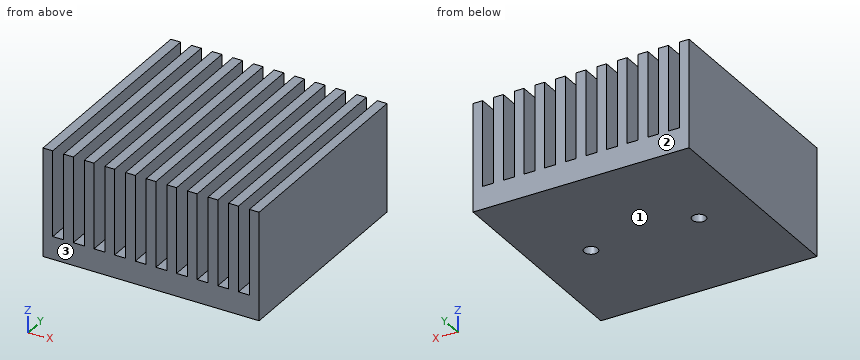
```python
from build123d import *

# Parameters (mm, degrees)
ESQUISSE1_W                = 40
ESQUISSE1_H                = 40
BOSS_EXTRU_1_DEPTH         = 4.2
ESQUISSE2_W                = 1.8
ESQUISSE2_H                = 15.8
BOSS_EXTRU_2_DEPTH         = 40
R_P_TITION_LIN_AIRE1_COUNT = 11
R_P_TITION_LIN_AIRE1_PITCH = 3.82
ESQUISSE3_R                = 1.25
ENL_V_MAT_EXTRU_1_DEPTH    = 10


with BuildPart() as part:
    # Esquisse1 → Boss.-Extru.1 (new body)
    with BuildSketch(Plane.XY):
        with Locations((20, 20)):
            Rectangle(ESQUISSE1_W, ESQUISSE1_H)
    extrude(amount=BOSS_EXTRU_1_DEPTH)

    # Esquisse2 → Boss.-Extru.2 (add)
    with BuildSketch(Plane.XZ):
        with Locations((0.9, 12.1)):
            Rectangle(ESQUISSE2_W, ESQUISSE2_H)
    boss_extru_2 = extrude(amount=-BOSS_EXTRU_2_DEPTH)

    # Répétition linéaire1: Boss.-Extru.2 ×11
    with Locations(*[(i * R_P_TITION_LIN_AIRE1_PITCH, 0, 0) for i in range(1, R_P_TITION_LIN_AIRE1_COUNT)]):
        add(boss_extru_2)

    # Esquisse3 → Enlèv. mat.-Extru.1 (cut)
    with BuildSketch(Plane(origin=(0, 0, 0), x_dir=(-1, 0, 0), z_dir=(0, 0, -1))):
        with Locations((-30, 20)):
            Circle(ESQUISSE3_R)
        with Locations((-10, 20)):
            Circle(ESQUISSE3_R)
    extrude(amount=-ENL_V_MAT_EXTRU_1_DEPTH, mode=Mode.SUBTRACT)


solid = part.part
```
The model under review builds one solid part; all positions refer to its coordinate system, in mm. Face numbers are marked on the shaded views. Give positions to 0.01 mm unless a question says otherwise; leave off trailing zeros. Loops run counter-clockwise (first coordinate to the right, second up) from the corner with the lowest first, then second, coordinate; pieces in that order, holes last. Notation, with made-up numbers: (4, 58.25) - (57, 58.25) arc R14 ccw to (57, 71.25) - close; hole circle Ø3 at (61, 21.25). An arc over 180 degrees is marked (long way). Answer as a JSON object with one key per item and string values.
Q1. Add section A-A on x = 10. State the section outline as (y, z) points, plus the area to 4 significant figures.
Worked out:
{"outline": "(0, 0) - (18.75, 0) - (18.75, 4.2) - (0, 4.2) - close; (21.25, 0) - (40, 0) - (40, 4.2) - (21.25, 4.2) - close", "area": "157.5 mm^2"}
Q2. To check wall thickness, follow line 1 along Z through (x, y) = (15, 28.5); line 2 along Y through (x, z) = (30, 3.5); line 3 along Y through (x, z) = (31, 5.5). State the ranges of each line that lie inside material, in increasing order.
Worked out:
{"line 1": "z = 0 to 4.2", "line 2": "y = 0 to 18.75, 21.25 to 40", "line 3": "y = 0 to 19.25, 20.75 to 40"}
Q3. Mouldability with a two-part tool opening along Y and no side actions: class the marked faces 1, 2 and 3 as +Y half, -Y half, draft (parallel to the pull), parting line (faces both ways), or undercut.
Worked out:
{"face 1": "draft", "face 2": "+Y half", "face 3": "-Y half"}
Q4. Add section B-B on y = 20. Count the separate pieces of the cut face and the enclosed holes in it, plus the area to 3 significant figures.
Worked out:
{"separate pieces": "3", "enclosed holes": "0", "area": "452 mm^2"}
Q5. Insertion check: pin 1 (3 mm diameter, centred on x = 12, y = 19.5, fed in from -Z); pin 2 (2 mm diameter, centred on x = 30, y = 20, fed in from -Z); pin 3 (0.6 mm diameter, centred on x = 14.5, y = 22.5, fed in from +Z). Each pin has a flat end and moves straight along its axis. Give the tip position at first contact, or say it passes through.
Worked out:
{"pin 1": "stops at z = 0", "pin 2": "stops at z = 10", "pin 3": "stops at z = 4.2"}
